```python
from build123d import *

# Parameters (mm, degrees)
F1_DEPTH = 44.45
F2_T     = -2.54
F3_R     = 5.08
F4_R     = 5.08
F5_W     = 19.812
F5_H     = 13.208
F6_DEPTH = 5.588
F7_W     = 15.24
F7_H     = 15.325371
F8_DEPTH = 6.604


with BuildPart() as f1:
    # F0 (on Top) → F1 (new body)
    with BuildSketch(Plane.XY):
        Polygon((-38.1, 27.86136), (-38.1, 1.19136), (-38.1, -25.47864), (44.45, -25.47864), (44.45, 1.19136), (44.45, 27.86136), align=None)
    extrude(amount=F1_DEPTH)

    # F2
    f2_openings = [f1.faces().sort_by_distance(p)[0] for p in [
        (3.175, 1.19136, 44.45),
    ]]
    offset(amount=F2_T, openings=f2_openings)

    # F3
    f3_edges = [f1.edges().sort_by_distance(p)[0] for p in [
        (-38.1, 27.86136, 22.225),
        (-38.1, -25.47864, 22.225),
        (44.45, -25.47864, 22.225),
        (44.45, 27.86136, 22.225),
    ]]
    fillet(f3_edges, radius=F3_R)

    # F4
    f4_edges = [f1.edges().sort_by_distance(p)[0] for p in [
        (3.175, 27.86136, 0),
        (42.962102, 26.373463, 0),
        (-36.612102, 26.373463, 0),
        (44.45, 1.19136, 0),
        (-38.1, 1.19136, 0),
        (42.962102, -23.990742, 0),
        (-36.612102, -23.990742, 0),
        (3.175, -25.47864, 0),
    ]]
    fillet(f4_edges, radius=F4_R)

    # F5 (on face) → F6 (cut)
    with BuildSketch(Plane.XZ.offset(25.47864)):
        with Locations((-23.114, 11.684)):
            Rectangle(F5_W, F5_H)
    extrude(amount=-F6_DEPTH, mode=Mode.SUBTRACT)

    # F7 (on face) → F8 (cut)
    with BuildSketch(Plane(origin=(0, 27.86136, 0), x_dir=(-1, 0, 0), z_dir=(0, 1, 0))):
        with Locations((25.4, 38.142685)):
            Rectangle(F7_W, F7_H)
    extrude(amount=-F8_DEPTH, mode=Mode.SUBTRACT)


solid = f1.part
```
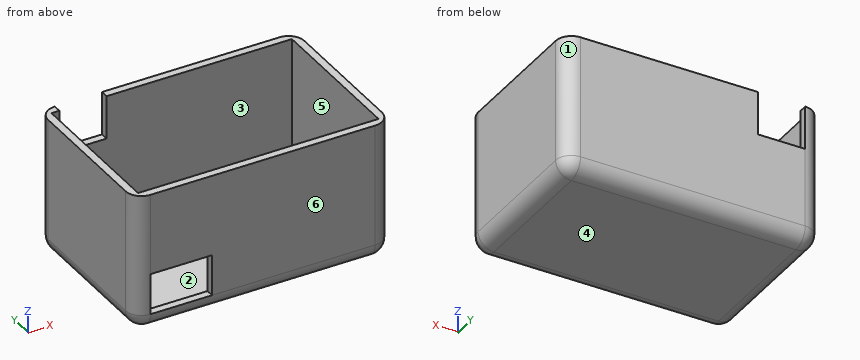
Source: CAD feature listing. Evaluate the final solid. Frame: model axes, mm. Face numbers are marked on the shaded views. A direction names the side the tool comes from. Round coordinates to 2 decimals unless told otherwise and drop trailing zeros. Write each loop counter-clockwise with the first axis right and the second up, starting at its lowest first coordinate (ties: lowest second). Pieces come first, ordered by that corner, then holes. Notation, with made-up numbers: M 47.25,17.25 L 76.25,17.25 A10 cw 76.25,28.25 Z; hole C 66.25,44.25 d1. An arc over 180 degrees is marked long. Answer as a JSON object with one key per item and string values. Group by question number.
(1) Ray query, line 1 (X direction, y = -14.5, z = 40); line 2 (Y direction, x = -13, z = 22); line 3 (Z direction, x = 29.5, y = -18). Return the intervals inside material, ascending. Write a range as [from, to].
(2) Section query D-D on y = -0.5. Output: boundary loops of the cut face in (x, z), then the cut area to 3 significant figures.
(3) Mould query, pull axis Y, two halves, no side actions, for the marked faces 1, 2, 3 and 4. Classes: +Y half, -Y half, draft (parallel to the pull), parting line (faces both ways), or undercut.
(4) First-contact query: pin 1 (1.3 mm diameter, centred on y = 26, z = 38, fed in from +X); pin 2 (2 mm diameter, centred on x = -26.5, y = 21.5, fed in from +Z); pin 3 (1.3 mm diameter, centred on x = -22, y = -24, fed in from -Z). Flat tips, straight axial feed; report the tip coordinate or a pass-through.
(5) Reachability of the marked faces 5 and 6 from +Z, -Z, +X, -X, +Y, -Y: full face, straight path, thin tool, end or side. Return the list, or none.
(6) Section query A-A on z = 29. Output: boundary loops of the cut face in (x, y), then the cut area to 3 significant figures.
(7) Section query C-C on z = 9.5. Output: boundary loops of the cut face in (x, y).
(8) Section query B-B on x = -22. Output: boundary loops of the cut face in (y, z), then the cut area to 3 significant figures.
Computed values:
{
 "1": {"line 1": "[-38.1, -35.56], [41.91, 44.45]", "line 2": "[-25.48, -22.94], [25.32, 27.86]", "line 3": "[0, 2.54]"},
 "2": {"outline": "M -38.1,5.08 A5.08 ccw -33.02,0 L 39.37,0 A5.08 ccw 44.45,5.08 L 44.45,44.45 L 41.91,44.45 L 41.91,2.54 L -35.56,2.54 L -35.56,44.45 L -38.1,44.45 Z", "area": "412 mm^2"},
 "3": {"face 1": "+Y half", "face 2": "undercut", "face 3": "undercut", "face 4": "draft"},
 "4": {"pin 1": "x = 43.75", "pin 2": "z = 2.54", "pin 3": "z = 0.95"},
 "5": {"face 5": "+Z", "face 6": "+Z, -Z, +X, -X, -Y"},
 "6": {"outline": "M -38.1,-20.4 A5.08 ccw -33.02,-25.48 L 39.37,-25.48 A5.08 ccw 44.45,-20.4 L 44.45,22.78 A5.08 ccw 39.37,27.86 L -33.02,27.86 A5.08 ccw -38.1,22.78 Z; hole M -35.56,-22.94 L 41.91,-22.94 L 41.91,25.32 L -35.56,25.32 Z", "area": "642 mm^2"},
 "7": {"outline": "M -38.1,-20.4 A5.08 ccw -33.02,-25.48 L -33.02,-22.94 L -35.56,-22.94 L -35.56,25.32 L 41.91,25.32 L 41.91,-22.94 L -13.21,-22.94 L -13.21,-25.48 L 39.37,-25.48 A5.08 ccw 44.45,-20.4 L 44.45,22.78 A5.08 ccw 39.37,27.86 L -33.02,27.86 A5.08 ccw -38.1,22.78 Z"},
 "8": {"outline": "M -25.48,5.08 A5.08 ccw -20.4,0 L 22.78,0 A5.08 ccw 27.86,5.08 L 27.86,30.48 L 25.32,30.48 L 25.32,2.54 L -22.94,2.54 L -22.94,5.08 Z; M -25.48,18.29 L -22.94,18.29 L -22.94,44.45 L -25.48,44.45 Z", "area": "268 mm^2"}
}
